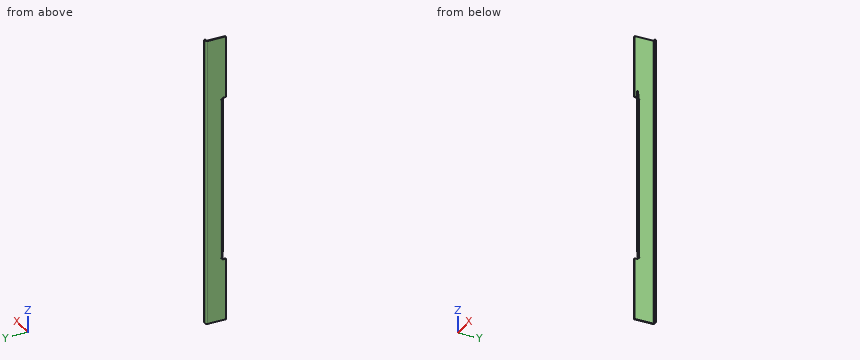
```python
from build123d import *

# Parameters (mm, degrees)
BASE_FLANGE1_DEPTH           = 3.175
EDGE_FLANGE1_START           = -833.4375
EDGE_FLANGE1_DEPTH           = 600.075
EDGE_FLANGE1_2_DEPTH         = 1.5875
EDGE_FLANGE1_START_2         = -234.95
EDGE_FLANGE1_3_DEPTH         = 1.5875
EDGE_FLANGE1_START_3         = -831.85
EDGE_FLANGE1_4_DEPTH         = 596.9
EDGE_FLANGE2_STRIP_W         = 19.05
EDGE_FLANGE2_STRIP_H         = 3.175
EDGE_FLANGE2_STRIP_CUT_DEPTH = 1066.8
EDGE_FLANGE2_DEPTH           = 1066.8


# Read off the part's stored shape, not the designer's step: Edge-Flange1
# Sheet-metal steps are written as plain solids
with BuildPart() as part:
    # Sketch1 → Base-Flange1 (new body)
    with BuildSketch(Plane(origin=(0, 0, 0), x_dir=(0, 0, -1), z_dir=(1, 0, 0))):
        Polygon((838.2, 0), (1066.8, 0), (1066.8, 73.025), (0, 73.025), (0, 0), (228.6, 0), (228.6, 12.7), (234.95, 12.7), (234.95, 11.43), (831.85, 11.43), (831.85, 12.7), (838.2, 12.7), align=None)
    extrude(amount=-BASE_FLANGE1_DEPTH)

    # Edge-Flange1 outline → Edge-Flange1 (cut)
    with BuildSketch(Plane.XY.offset(EDGE_FLANGE1_START)):
        with BuildLine():
            Line((-3.175, 16.929261314), (-3.175, 11.43))
            Line((-3.175, 11.43), (0, 11.43))
            ThreePointArc((0, 11.43), (-2.324261314, 13.754261314), (-3.175, 16.929261314))
        make_face()
    extrude(amount=EDGE_FLANGE1_DEPTH, mode=Mode.SUBTRACT)

    # Edge-Flange1 2 outline → Edge-Flange1 2 (cut)
    with BuildSketch(Plane.XY.offset(EDGE_FLANGE1_START)):
        with BuildLine():
            Line((0, 18.516761314), (-3.175, 18.516761314))
            Line((-3.175, 18.516761314), (-3.175, 16.929261314))
            ThreePointArc((-3.175, 16.929261314), (-2.757968249, 14.665992052), (-1.561649527, 12.7))
            Line((-1.561649527, 12.7), (0, 12.7))
            Line((0, 12.7), (0, 18.516761314))
        make_face()
    extrude(amount=EDGE_FLANGE1_2_DEPTH, mode=Mode.SUBTRACT)

    # Edge-Flange1 3 outline → Edge-Flange1 3 (cut)
    with BuildSketch(Plane.XY.offset(EDGE_FLANGE1_START_2)):
        with BuildLine():
            Line((0, 18.516761314), (-3.175, 18.516761314))
            Line((-3.175, 18.516761314), (-3.175, 16.929261314))
            ThreePointArc((-3.175, 16.929261314), (-2.757968249, 14.665992052), (-1.561649527, 12.7))
            Line((-1.561649527, 12.7), (0, 12.7))
            Line((0, 12.7), (0, 18.516761314))
        make_face()
    extrude(amount=EDGE_FLANGE1_3_DEPTH, mode=Mode.SUBTRACT)

    # Edge-Flange1 4 outline → Edge-Flange1 4 (add)
    with BuildSketch(Plane.XY.offset(EDGE_FLANGE1_START_3)):
        with BuildLine():
            ThreePointArc((1.5875, 14.179630657), (0.425369343, 15.341761314), (0, 16.929261314))
            Line((0, 16.929261314), (0, 11.43))
            Line((0, 11.43), (46.318351826, -15.311912895))
            Line((46.318351826, -15.311912895), (47.905851826, -12.562282238))
            Line((47.905851826, -12.562282238), (1.5875, 14.179630657))
        make_face()
    extrude(amount=EDGE_FLANGE1_4_DEPTH)

    # Edge-Flange2 strip (across the edge) → Edge-Flange2 strip cut (cut)
    with BuildSketch(Plane(origin=(0, 73.025, -1066.8), x_dir=(0, -1, 0), z_dir=(0, 0, 1))):
        with Locations((-3.175, -1.5875)):
            Rectangle(EDGE_FLANGE2_STRIP_W, EDGE_FLANGE2_STRIP_H)
    extrude(amount=EDGE_FLANGE2_STRIP_CUT_DEPTH, mode=Mode.SUBTRACT)

    # Edge-Flange2 section (across the edge) → Edge-Flange2 (add)
    with BuildSketch(Plane(origin=(0, 73.025, -1066.8), x_dir=(0, -1, 0), z_dir=(0, 0, 1))):
        with BuildLine():
            Line((0, 3.175), (0, 9.525))
            Line((0, 9.525), (3.175, 9.525))
            Line((3.175, 9.525), (3.175, 3.175))
            ThreePointArc((3.175, 3.175), (4.10493597, 0.92993597), (6.35, 0))
            Line((6.35, 0), (6.35, -3.175))
            ThreePointArc((6.35, -3.175), (1.859871939, -1.315128061), (0, 3.175))
        make_face()
    extrude(amount=EDGE_FLANGE2_DEPTH)


solid = part.part
```
Geometry: final body of the model. Coordinates: model frame, mm. Coordinates: 2 decimals unless noted, no trailing zeros. Write each loop counter-clockwise with the first axis right and the second up, starting at its lowest first coordinate (ties: lowest second). Pieces come first, ordered by that corner, then holes. Notation, with made-up numbers: M 6.5,3 L 18.5,3 A15 ccw 18.5,26 Z; hole C 9,-6.75 d7. An arc over 180 degrees is marked long. Use CSV: the item, a comma, the result in double quotes. Start each with the question number.
1. Cut plane D-D on x = 29.5. Return the cut outline in (y, z).
2. Cut plane B-B on y = 53.5. Return the cut outline in (x, z) (3 decimals).
3. First-contact query: P1, Ø1.7, axis at x = -1.5, z = -833, coming from the -Y side; P2, Ø3, axis at y = 3.5, z = -430.5, coming from the +X side; P3, Ø1, axis at y = 43.5, z = -943.5, coming from the +X side; P4, Ø3.5, axis at x = -2, y = 5, coming from the +Z side. Flat tips, straight axial feed; report the tip coordinate or a pass-through.
4. Ray query, probe 1 along X at (y, z) = (25.5, -763.5) (3 decimals); probe 2 along Y at (x, z) = (7.5, -261.5) (3 decimals); probe 3 along Y at (x, z) = (6, -720) (3 decimals). Return the intervals inside material, ascending.
5. Cut plane A-A on z = -131.5. Return the cut outline in (x, y) (3 decimals).
Entries:
1,outline,"M -5.6,-831.85 L -1.94,-831.85 L -1.94,-234.95 L -5.6,-234.95 Z"
2,outline,"M -3.175,-1066.8 L 0,-1066.8 L 0,0 L -3.175,0 Z"
3,P1,"y = 12.7"
3,P2,"x = 22.68"
3,P3,"x = 0"
3,P4,"z = 0"
4,probe 1,"-3.175 to 0"
4,probe 2,"7.1 to 10.766, 69.85 to 73.025"
4,probe 3,"7.966 to 11.632, 69.85 to 73.025"
5,outline,"M -3.175,0 L 0,0 L 0,66.675 A3.175 cw 3.175,69.85 L 9.525,69.85 L 9.525,73.025 L 3.175,73.025 A6.35 ccw -3.175,66.675 Z"
